from build123d import *

# Parameters (mm, degrees)
SKETCH_1_R      = 40
EXTRUDE_1_DEPTH = 44
SKETCH_3_R      = 12.5
EXTRUDE_2_DEPTH = 84
CHAMFER_1_SIZE  = 6
CHAMFER_1_SIZE2 = 10.392304845


with BuildPart() as part:
    # 草图1 → 凸台-拉伸1 (new body)
    with BuildSketch(Plane(origin=(0, 0, 0), x_dir=(1, 0, 0), z_dir=(0, 1, 0))):
        with Locations(Location((0, 0, 0), (0, 0, 270))):
            Circle(SKETCH_1_R)
    extrude(amount=EXTRUDE_1_DEPTH)

    # 草图3 → 凸台-拉伸2 (add)
    with BuildSketch(Plane.XZ):
        with Locations(Location((0, 0, 0), (0, 0, 270))):
            Circle(SKETCH_3_R)
    extrude(amount=-EXTRUDE_2_DEPTH)

    # 倒角1
    chamfer_1_edges = [part.edges().sort_by_distance(p)[0] for p in [
        (0, 84, 12.5),
    ]]
    chamfer_1_side = [part.faces().sort_by_distance(p)[0] for p in [
        (0, 84, 0),
    ]]
    chamfer(chamfer_1_edges, length=CHAMFER_1_SIZE, length2=CHAMFER_1_SIZE2, reference=chamfer_1_side[0])


solid = part.part
The model under review builds one solid part; all positions refer to its coordinate system, in mm. A direction names the side the tool comes from. Round coordinates to 2 decimals unless told otherwise and drop trailing zeros. Order: outer loops, then holes, each group sorted by start corner. A loop starts at its lowest first (then second) coordinate and runs counter-clockwise, first axis right, second up. Notation, with made-up numbers: (52, -30.5) - (74, -30.5) arc R18 ccw to (74, 4.5) - close; hole circle Ø9 at (-4.75, 5.5). An arc over 180 degrees is marked (long way). Use one line per item in the form item = value.
Q1. Tool access review of faces 1 (the flat face through (9, 44, -9)), 2 (the cylindrical face through (-39.05, 21.69, -8.67)): name each direction out of +Z, -Z, +X, -X, +Y, -Y from which nothing blocks a thin tool from reaching the whole face with its end or side.
Response values:
face_1 = +Y
face_2 = +Y, -Y
Q2. Add section D-D on x = -26.5. Give the boundary of the cut face in (y, z).
Response values:
outline = (0, -29.96) - (44, -29.96) - (44, 29.96) - (0, 29.96) - close
Q3. Add section A-A on z = 0. Give the boundary of the cut face in (x, y).
Response values:
outline = (-40, 0) - (40, 0) - (40, 44) - (12.5, 44) - (12.5, 73.61) - (6.5, 84) - (-6.5, 84) - (-12.5, 73.61) - (-12.5, 44) - (-40, 44) - close
Q4. Clearance check with flat-ended pins moving along their axes: P1, Ø3, axis at x = 16, z = -17, coming from the +Y side; P2, Ø12, axis at x = 4.5, z = -16.5, coming from the +Y side; P3, Ø8, axis at y = 32.5, z = 23.5, coming from the -X side. State where each tip first meets the part, or that it passes through.
Response values:
P1 = 44
P2 = 76.03
P3 = -34.92
Q5. To check wall thickness, follow line 1 (Y direction, x = 20, z = 9.5); line 2 (X direction, y = 28, z = -34); line 3 (X direction, y = 11.5, z = -33). State the ranges of each line that lie inside material, in increasing order.
Response values:
line_1 = 0 to 44
line_2 = -21.07 to 21.07
line_3 = -22.61 to 22.61
Q6. Add section B-B on x = 0. Give the boundary of the cut face in (y, z), then the cut area to 3 significant figures.
Response values:
outline = (0, -40) - (44, -40) - (44, -12.5) - (73.61, -12.5) - (84, -6.5) - (84, 6.5) - (73.61, 12.5) - (44, 12.5) - (44, 40) - (0, 40) - close
area = 4,460 mm^2
Q7. Add section C-C on y = 23.5. Give the boundary of the cut face in (x, z).
Response values:
outline = circle Ø80 at (0, 0)
